from build123d import *

# Parameters (mm, degrees)
SKETCH1_W           = 120
SKETCH1_H           = 26
BOSS_EXTRUDE1_DEPTH = 25
SKETCH3_W           = 84
SKETCH3_H           = 26
CUT_EXTRUDE1_DEPTH  = 20
SKETCH4_W           = 10
SKETCH4_H           = 26
CUT_EXTRUDE2_DEPTH  = 5
CHAMFER1_SIZE       = 5
SKETCH5_W           = 20.1
SKETCH5_H           = 20.1
CUT_EXTRUDE3_DEPTH  = 20
FILLET1_R           = 5
FILLET2_R           = 2
CUT_EXTRUDE4_DEPTH  = 30


with BuildPart() as part:
    # Sketch1 → Boss-Extrude1 (new body)
    with BuildSketch(Plane(origin=(0, 0, 0), x_dir=(1, 0, 0), z_dir=(0, 1, 0))):
        Rectangle(SKETCH1_W, SKETCH1_H)
    extrude(amount=BOSS_EXTRUDE1_DEPTH)

    # Sketch3 → Cut-Extrude1 (cut)
    with BuildSketch(Plane(origin=(0, 25, 0), x_dir=(1, 0, 0), z_dir=(0, 1, 0))):
        with Locations((-8, 0)):
            Rectangle(SKETCH3_W, SKETCH3_H)
    extrude(amount=-CUT_EXTRUDE1_DEPTH, mode=Mode.SUBTRACT)

    # Sketch4 → Cut-Extrude2 (cut)
    with BuildSketch(Plane(origin=(0, 25, 0), x_dir=(1, 0, 0), z_dir=(0, 1, 0))):
        with Locations((-55, 0)):
            Rectangle(SKETCH4_W, SKETCH4_H)
    extrude(amount=-CUT_EXTRUDE2_DEPTH, mode=Mode.SUBTRACT)

    # Chamfer1
    chamfer1_edges = [part.edges().sort_by_distance(p)[0] for p in [
        (-50, 5, 0),
        (34, 5, 0),
    ]]
    chamfer(chamfer1_edges, length=CHAMFER1_SIZE)

    # Sketch5 → Cut-Extrude3 (cut)
    with BuildSketch(Plane(origin=(0, 25, 0), x_dir=(1, 0, 0), z_dir=(0, 1, 0))):
        with Locations((47, 0)):
            Rectangle(SKETCH5_W, SKETCH5_H)
    extrude(amount=-CUT_EXTRUDE3_DEPTH, mode=Mode.SUBTRACT)

    # Fillet1
    fillet1_edges = [part.edges().sort_by_distance(p)[0] for p in [
        (60, 0, 0),
        (-60, 0, 0),
    ]]
    fillet(fillet1_edges, radius=FILLET1_R)

    # Fillet2
    fillet2_edges = [part.edges().sort_by_distance(p)[0] for p in [
        (-60, 12.5, -13),
        (-60, 12.5, 13),
        (-8, 5, 13),
        (-8, 5, -13),
        (-50, 15, 13),
        (-50, 15, -13),
        (34, 17.5, -13),
        (34, 17.5, 13),
        (-47.5, 7.5, 13),
        (-47.5, 7.5, -13),
        (31.5, 7.5, -13),
        (31.5, 7.5, 13),
        (0, 0, -13),
        (-58.535533906, 1.464466094, -13),
        (58.535533906, 1.464466094, -13),
        (0, 0, 13),
        (-58.535533906, 1.464466094, 13),
        (58.535533906, 1.464466094, 13),
        (60, 15, -13),
        (60, 15, 13),
    ]]
    fillet(fillet2_edges, radius=FILLET2_R)

    # Sketch6 → Cut-Extrude4 (cut)
    with BuildSketch(Plane(origin=(60, 0, 0), x_dir=(0, 0, -1), z_dir=(1, 0, 0))):
        with BuildLine():
            Line((3, 17.5), (3, 12.5))
            ThreePointArc((3, 12.5), (0, 9.5), (-3, 12.5))
            Line((-3, 12.5), (-3, 17.5))
            ThreePointArc((-3, 17.5), (0, 20.5), (3, 17.5))
        make_face()
    extrude(amount=-CUT_EXTRUDE4_DEPTH, mode=Mode.SUBTRACT)


solid = part.part
Source: CAD feature listing. Evaluate the final solid. Frame: model axes, mm. A direction names the side the tool comes from. Coordinates: 2 decimals unless noted, no trailing zeros. Loops run counter-clockwise (first coordinate to the right, second up) from the corner with the lowest first, then second, coordinate; pieces in that order, holes last. Notation, with made-up numbers: (-19.75, -0.75) -> (2.25, -0.75) arc R7 cw to (2.25, 9.25) -> close; hole circle Ø9 at (28, 34.5). An arc over 180 degrees is marked (long way). Answer in a Markdown table with one row per item. Add a question column.
Q1. Section B-B on z = 0. Return the cut outline in (x, y), and give its area (3 significant figures).
Q2. Reachability of faces 1 (the face through (47, 5, 0)), 2 (the face through (58.5, 9.5, -0.1)), 3 (the face through (-9, 5, 0)), 4 (the face through (-7.47, 4.4, -12.43)) from +Z, -Z, +X, -X, +Y, -Y: full face, straight path, thin tool, end or side. Return the list, or none.
Q3. Contact query for flat-ended pins moving along their axis: pin 1 Ø1.5 at (x, y) = (35, 15) entering from +Z; pin 2 Ø5 at (y, z) = (19, 2.5) entering from +X; pin 3 Ø8 at (x, z) = (-53.5, 2) entering from +Y; pin 4 Ø8 at (x, z) = (27, -7) entering from +Y. Output: stop coordinate, or through.
Q4. Pull-direction query (Z, two-part tool) for faces 5 (the face through (-0.77, 0.6, -12.43)), 6 (the face through (-60, 12, 0)), 7 (the face through (47, 15, -10.05)); classes: pulls with the +Z half, pulls with the -Z half, needs draft (parallel to the pull), parting line crosses it, or undercut.
Q5. Section C-C on x = -30.5. Return the cut outline in (y, z), and give its area (3 significant figures).
Q6. Section D-D on z = 9. Return the cut outline in (x, y), and give its area (3 significant figures).
Q7. Ray query, line 1 along X through (y, z) = (11.75, -5); line 2 along Z through (x, y) = (44.5, 15); line 3 along X through (y, z) = (15, -11.25). Return the intervals inside material, ascending.
Q8. Section A-A on y = 15. Return the cut outline in (x, z).
Computed values:
| question | item | result |
|---|---|---|
| 1 | outline | (-60, 5) arc R5 ccw to (-55, 0) -> (55, 0) arc R5 ccw to (60, 5) -> (60, 9.5) -> (57.05, 9.5) -> (57.05, 5) -> (36.95, 5) -> (36.95, 9.5) -> (33.5, 9.5) -> (29, 5) -> (-45, 5) -> (-50, 10) -> (-50, 20) -> (-60, 20) -> close; (34, 20.5) -> (36.95, 20.5) -> (36.95, 25) -> (34, 25) -> close; (57.05, 20.5) -> (60, 20.5) -> (60, 25) -> (57.05, 25) -> close |
| 1 | area | 817 mm^2 |
| 2 | face 1 | +Y |
| 2 | face 2 | +X |
| 2 | face 3 | +Z, -Z, +Y |
| 2 | face 4 | -Z, +Y |
| 3 | pin 1 | stops at z = 12.98 |
| 3 | pin 2 | stops at x = 60 |
| 3 | pin 3 | stops at y = 20 |
| 3 | pin 4 | stops at y = 7 |
| 4 | face 5 | pulls with the -Z half |
| 4 | face 6 | needs draft |
| 4 | face 7 | undercut |
| 5 | outline | (0, -11) arc R2 ccw to (2, -13) -> (3, -13) arc R2 ccw to (5, -11) -> (5, 11) arc R2 ccw to (3, 13) -> (2, 13) arc R2 ccw to (0, 11) -> close |
| 5 | area | 127 mm^2 |
| 6 | outline | (-60, 5) arc R5 ccw to (-55, 0) -> (55, 0) arc R5 ccw to (60, 5) -> (60, 25) -> (57.05, 25) -> (57.05, 5) -> (36.95, 5) -> (36.95, 25) -> (34, 25) -> (34, 10) -> (29, 5) -> (-45, 5) -> (-50, 10) -> (-50, 20) -> (-60, 20) -> close |
| 6 | area | 882 mm^2 |
| 7 | line 1 | x = -60 to -50, 34 to 36.95, 57.05 to 60 |
| 7 | line 2 | z = -13 to -10.05, 10.05 to 13 |
| 7 | line 3 | x = -59.98 to -50.02, 34.02 to 59.98 |
| 8 | outline | (-60, -11) arc R2 ccw to (-58, -13) -> (-52, -13) arc R2 ccw to (-50, -11) -> (-50, 11) arc R2 ccw to (-52, 13) -> (-58, 13) arc R2 ccw to (-60, 11) -> close; (34, -11) arc R2 ccw to (36, -13) -> (58, -13) arc R2 ccw to (60, -11) -> (60, -3) -> (57.05, -3) -> (57.05, -10.05) -> (36.95, -10.05) -> (36.95, -3) -> (34, -3) -> close; (34, 3) -> (36.95, 3) -> (36.95, 10.05) -> (57.05, 10.05) -> (57.05, 3) -> (60, 3) -> (60, 11) arc R2 ccw to (58, 13) -> (36, 13) arc R2 ccw to (34, 11) -> close |
